from build123d import *

# Parameters (mm, degrees)
F0_W     = 25
F0_H     = 30
F1_DEPTH = 12.5
F2_W     = 20
F2_H     = 20
F3_DEPTH = 20
F4_R     = 3.175
F5_DEPTH = 25.001
F6_R     = 2


with BuildPart() as f1:
    # F0 (on Front) → F1 (new body, symmetric)
    with BuildSketch(Plane.XZ):
        with Locations((12.5, 15)):
            Rectangle(F0_W, F0_H)
    extrude(amount=F1_DEPTH, both=True)

    # F2 (on face) → F3 (cut)
    with BuildSketch(Plane(origin=(0, 12.5, 0), x_dir=(-1, 0, 0), z_dir=(0, 1, 0))):
        with Locations((-15, 15)):
            Rectangle(F2_W, F2_H)
    extrude(amount=-F3_DEPTH, mode=Mode.SUBTRACT)

    # F4 (on face) → F5 (cut, through all)
    with BuildSketch(Plane(origin=(0, 0, 0), x_dir=(0, -1, 0), z_dir=(-1, 0, 0))):
        with Locations((-2.5, 15)):
            Circle(F4_R)
    extrude(amount=-F5_DEPTH, mode=Mode.SUBTRACT)

    # F6
    f6_edges = [f1.edges().sort_by_distance(p)[0] for p in [
        (0, 0, 30),
        (12.5, 12.5, 30),
        (12.5, -12.5, 30),
        (25, 0, 30),
        (0, -12.5, 15),
        (12.5, -12.5, 0),
        (25, -12.5, 15),
        (0, 0, 0),
        (12.5, 12.5, 0),
        (25, 0, 0),
        (0, 12.5, 15),
    ]]
    fillet(f6_edges, radius=F6_R)


solid = f1.part
Geometry: final body of the model. Coordinates: model frame, mm. A direction names the side the tool comes from. Round coordinates to 2 decimals unless told otherwise and drop trailing zeros. Loops run counter-clockwise (first coordinate to the right, second up) from the corner with the lowest first, then second, coordinate; pieces in that order, holes last. Notation, with made-up numbers: (76, 25.5) -> (134, 25.5) arc R20 ccw to (134, 31.5) -> close; hole circle Ø3 at (-21, -15.5). An arc over 180 degrees is marked (long way). One line per question, with ' | ' between items. Start each with the question number.
1. Section C-C on x = 19. Output: boundary loops of the cut face in (y, z), and give its area (3 significant figures).
2. Section D-D on y = -6.5. Output: boundary loops of the cut face in (x, z), and give its area (3 significant figures).
3. Section B-B on z = 15. Output: boundary loops of the cut face in (x, y) (3 decimals).
4. Contact query for flat-ended pins moving along their axis: pin 1 (5 mm diameter, centred on x = 17.5, z = 19, fed in from +Y); pin 2 (12 mm diameter, centred on y = 8.5, z = 11.5, fed in from +X). Output: stop coordinate, or through.
5. Set-up query: faces 4 (the face through (2.46, 2.91, 18.15)), 5 (the face through (15, -7.5, 15)). Return all of +Z, -Z, +X, -X, +Y, -Y with unobstructed straight access to the full face (end or side cutting, diameter ignored); none if empty.
6. Section A-A on y = 2.5. Output: boundary loops of the cut face in (x, z) (3 decimals).
7. Mould query, pull axis Z, two halves, no side actions, for faces 1 (the face through (0.57, -0.15, 0.6)), 2 (the face through (0.57, -11.9, 15.18)), 3 (the face through (15, 3, 5)). Classes: pulls with the +Z half, pulls with the -Z half, needs draft (parallel to the pull), parting line crosses it, or undercut.
8. Line query: line 1 along Z through (x, y) = (2.75, 2.5) (3 decimals); line 2 along Z through (x, y) = (20.25, 0.75); line 3 along Y through (x, z) = (21.5, 6.25). Output: solid intervals per line, ascending. Write a range as [from, to].
Returned:
1) outline: (-12.5, 2) arc R2 ccw to (-10.5, 0) -> (10.5, 0) arc R2 ccw to (12.5, 2) -> (12.5, 5) -> (-7.5, 5) -> (-7.5, 25) -> (12.5, 25) -> (12.5, 28) arc R2 ccw to (10.5, 30) -> (-10.5, 30) arc R2 ccw to (-12.5, 28) -> close | area: 347 mm2
2) outline: (0, 2) arc R2 ccw to (2, 0) -> (23, 0) arc R2 ccw to (25, 2) -> (25, 5) -> (5, 5) -> (5, 25) -> (25, 25) -> (25, 28) arc R2 ccw to (23, 30) -> (2, 30) arc R2 ccw to (0, 28) -> close | area: 347 mm2
3) outline: (0, -10.5) arc R2 ccw to (2, -12.5) -> (23, -12.5) arc R2 ccw to (25, -10.5) -> (25, -7.5) -> (5, -7.5) -> (5, -0.675) -> (0, -0.675) -> close; (0, 5.675) -> (5, 5.675) -> (5, 12.5) -> (2, 12.5) arc R2 ccw to (0, 10.5) -> close
4) pin 1: stops at y = -7.5 | pin 2: stops at x = 5
5) face 4: +X, -X | face 5: +X, +Y
6) outline: (0, 2) arc R2 ccw to (2, 0) -> (23, 0) arc R2 ccw to (25, 2) -> (25, 5) -> (5, 5) -> (5, 11.825) -> (0, 11.825) -> close; (0, 18.175) -> (5, 18.175) -> (5, 25) -> (25, 25) -> (25, 28) arc R2 ccw to (23, 30) -> (2, 30) arc R2 ccw to (0, 28) -> close
7) face 1: pulls with the -Z half | face 2: needs draft | face 3: undercut
8) line 1: z = [0, 11.825], [18.175, 30] | line 2: z = [0, 5], [25, 30] | line 3: y = [-12.5, -7.5]
